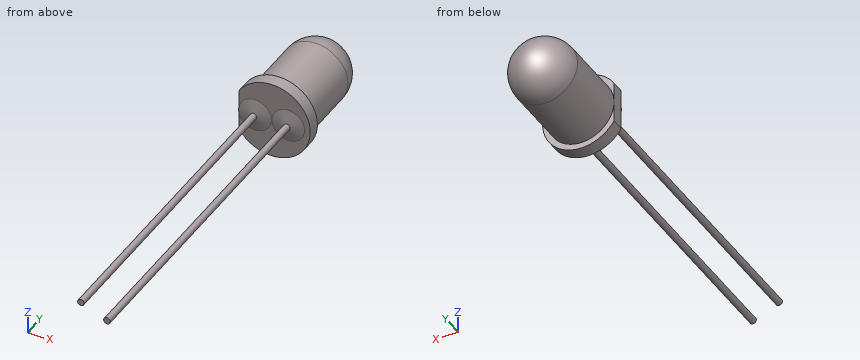
Autodesk Inventor part; units mm, degrees
ref_plane "Work Plane1" through (1.27, -28.95, 0) normal (0, -1, 0) x (1, 0, 0)
ref_plane "Work Plane2" through (-1.27, -27.95, 0) normal (0, -1, 0) x (1, 0, 0)
ref_plane "YZ Plane" through (0, 0, 0) normal (1, 0, 0) x (0, 1, 0)
sketch "Sketch1" plane through (0, 0, 0) normal (0, 0, 1) x (1, 0, 0)
  line L0 (2.5, -2.55) -> (-2.5, -2.55)
  line L1 (-2.5, -2.55) -> (-2.5, 2.55)
  line L2 (-2.5, 2.55) -> (2.5, 2.55)
  line L3 (2.5, 2.55) -> (2.5, -2.55)
  line L4 (2.5, -2.55) -> (-2.5, 2.55) construction
  line L5 (-2.5, -2.55) -> (2.5, 2.55) construction
  arc A0 (2.5, 2.55) -> (-2.5, 2.55) centre (0, 2.55) ccw
  line L6 (-2.95, -2.55) -> (2.95, -2.55)
  line L7 (2.95, -2.55) -> (2.95, -3.55)
  line L8 (2.95, -3.55) -> (-2.95, -3.55)
  line L9 (-2.95, -3.55) -> (-2.95, -2.55)
  line L10 (0, 5.05) -> (0, -3.55)
  point P0 (0, 0)
  point P1 (0, -2.55)
  point P2 (0, -2.55)
  dimension "d0" = 5
  dimension "d1" = 1
  dimension "d2" = 5.9
  dimension "d3" = 8.6
revolve "Revolution1" add sketch "Sketch1" angle 360 about axis through (0, 5.05, 0) along (0, -1, 0) picked at (1.5632, 3.097) contours L6 L7 L8 L10 L0 | L0 L10 L2 L3 | L2 L10 A0
sketch "Sketch2" plane through (0, 0, 0) normal (0, 0, 1) x (1, 0, 0)
  line L0 (-2.95, -3.55) -> (2.95, -3.55)
  line L1 (-1.27, -3.55) -> (-1.27, -27.95)
  line L2 (1.27, -3.55) -> (1.27, -28.95)
  line L3 (-2.95, -2.55) -> (-2.95, -3.55)
  line L4 (-2.95, -2.55) -> (2.95, -2.55)
  line L5 (-2.5, 2.55) -> (-2.5, -2.55)
  line L6 (-2.5, -2.55) -> (-2.5, -3.55)
  point P0 (0, 0)
  point P1 (0, -3.55)
  dimension "d5" = 2.54
  dimension "d6" = 1.27
  dimension "d7" = 25.4
  dimension "d8" = 1
ref_plane "Work Plane1" through (1.27, -28.95, 0) normal (0, -1, 0) x (1, 0, 0)
ref_plane "Work Plane2" through (-1.27, -27.95, 0) normal (0, -1, 0) x (1, 0, 0)
sketch "Sketch3" plane through (1.27, -28.95, 0) normal (0, -1, 0) x (1, 0, 0)
  circle A0 centre (0, 0) radius 0.25
  circle A1 centre (-2.54, 0) radius 0.25
  point P0 (-1.27, 0)
  dimension "d9" = 0.5
extrude "Extrusion1" add sketch "Sketch3" against normal up to surface (25.4 mm away) contours A0
extrude "Extrusion2" add sketch "Sketch3" against normal up to surface (24.4 mm away) from surface at -1 contours A1
chamfer "Chamfer1" distance 1 distance2 0.2 1 edges at (-1.52, -3.55, 0) measured on face at (0.1185, -3.55, -1.0867)
chamfer "Chamfer2" distance 1 distance2 0.2 1 edges at (1.02, -3.55, 0) measured on face at (0.8409, -3.55, -1.1635)
extrude "Extrusion3" cut sketch "Sketch2" along normal through all both and the other way through all
properties part number "5mm_LED_Red"
The listing builds one solid part. Answer for the finished solid, in the listing's coordinates (mm). Coordinates: 2 decimals unless noted, no trailing zeros. Write each loop counter-clockwise with the first axis right and the second up, starting at its lowest first coordinate (ties: lowest second). Pieces come first, ordered by that corner, then holes. Notation, with made-up numbers: (16.5, -34) - (69.5, -34) arc R26 cw to (69.5, -8) - close; hole circle Ø5 at (86, 87). An arc over 180 degrees is marked (long way). Put each result on its own line as item: value.
1. Flat-ended cylindrical pins translate along their axes: pin 1 Ø1 at (x, z) = (1, 2.5) entering from +Y; pin 2 Ø1.5 at (x, z) = (-1, -1) entering from +Y; pin 3 Ø0.5 at (y, z) = (-3, 0) entering from -X. Find the tip coordinate at first contact, or state that the pin passes through.
Answer sheet:
pin 1: stops at y = 3.75
pin 2: stops at y = 4.96
pin 3: stops at x = -2.5
2. Find the intervals of material crossed by line 1 along Y through (x, z) = (-1.5, -2.25); line 2 along Z through (x, y) = (1.3, -23); line 3 along Y through (x, z) = (-1.8, 0.5), in increasing order. Write a range as from..to.
Answer sheet:
line 1: y = -3.55..-2.55
line 2: z = -0.25..0.25
line 3: y = -3.65..4.21
3. The part is cut by section A-A on y = -11. Give the vertices of the cut face in (x, z), plus the area to 3 significant figures.
Answer sheet:
outline: circle Ø0.5 at (-1.27, 0); circle Ø0.5 at (1.27, 0)
area: 0.393 mm^2
